Verification items for the finished model (mm, model axes). Face numbers are marked on the shaded views. A direction names the side the tool comes from. Round coordinates to 2 decimals unless told otherwise and drop trailing zeros. Loops run counter-clockwise (first coordinate to the right, second up) from the corner with the lowest first, then second, coordinate; pieces in that order, holes last. Notation, with made-up numbers: (-15, 26.5) - (17, 26.5) arc R6 ccw to (17, 32.5) - close; hole circle Ø7 at (-20, -0.5). An arc over 180 degrees is marked (long way). Use CSV: the item, a comma, the result in double quotes.
```python
from build123d import *

# Parameters (mm, degrees)
SKETCH1_R           = 3.3
BOSS_EXTRUDE1_DEPTH = 10
CUT_EXTRUDE1_DEPTH  = 5


with BuildPart() as part:
    # Sketch1 → Boss-Extrude1 (new body)
    with BuildSketch(Plane(origin=(0, 0, 0), x_dir=(1, 0, 0), z_dir=(0, 1, 0))):
        with BuildLine():
            Line((10, 0), (10, -10))
            ThreePointArc((10, -10), (0, -20), (-10, -10))
            Line((-10, -10), (-10, 0))
            ThreePointArc((-10, 0), (0, 10), (10, 0))
        make_face()
        with Locations(Location((0, 0, 0), (0, 0, 270))):
            Circle(SKETCH1_R, mode=Mode.SUBTRACT)
    extrude(amount=BOSS_EXTRUDE1_DEPTH)

    # Sketch2 → Cut-Extrude1 (cut)
    with BuildSketch(Plane.XZ):
        Polygon((6.5, 3.75277675), (0, 7.505553499), (-6.5, 3.75277675), (-6.5, -3.75277675), (0, -7.505553499), (6.5, -3.75277675), align=None)
    extrude(amount=-CUT_EXTRUDE1_DEPTH, mode=Mode.SUBTRACT)


solid = part.part
```
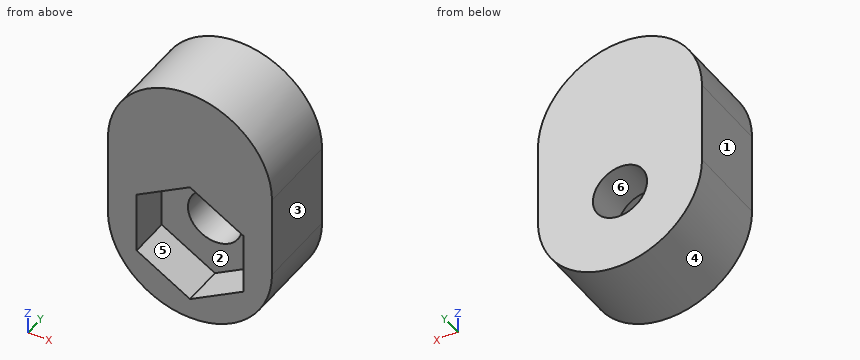
1) Access from +Z, -Z, +X, -X, +Y, -Y to the whole of each face (thin tool, end or side, straight path). Record for the marked faces 5 and 6.
Returned:
face 5,"-Y"
face 6,"+Y, -Y"
2) Mould release check, pull along X, two halves, no side actions. Record for the marked faces 1, 2, 3 and 4: +X half, -X half, draft (parallel to the pull), parting line (faces both ways), or undercut.
Returned:
face 1,"-X half"
face 2,"undercut"
face 3,"+X half"
face 4,"parting line"
3) Cross-section at D-D, the plane x = 4.25. Record the cut outline in (y, z), then the cut area to 3 significant figures.
Returned:
outline,"(0, -9.05) - (10, -9.05) - (10, 19.05) - (0, 19.05) - (0, 5.05) - (5, 5.05) - (5, -5.05) - (0, -5.05) - close"
area,"231 mm²"
4) Thickness scan on probe 1 along X at (y, z) = (6, 0); probe 2 along Z at (x, y) = (0, 8.7); probe 3 along Y at (x, z) = (0.75, -6). Record the ranges inside material, lowest first. Write a range as [from, to].
Returned:
probe 1,"x = [-10, -3.3], [3.3, 10]"
probe 2,"z = [-10, -3.3], [3.3, 20]"
probe 3,"y = [5, 10]"
5) Cross-section at A-A, the plane y = 3.75. Record the cut outline in (x, z).
Returned:
outline,"(-10, 0) arc R10 ccw to (10, 0) - (10, 10) arc R10 ccw to (-10, 10) - close; hole (-6.5, -3.75) - (0, -7.51) - (6.5, -3.75) - (6.5, 3.75) - (0, 7.51) - (-6.5, 3.75) - close"
6) Cross-section at B-B, the plane x = -2.5. Record the cut outline in (y, z), then the cut area to 3 significant figures.
Returned:
outline,"(0, -9.68) - (10, -9.68) - (10, -2.15) - (5, -2.15) - (5, -6.06) - (0, -6.06) - close; (0, 6.06) - (5, 6.06) - (5, 2.15) - (10, 2.15) - (10, 19.68) - (0, 19.68) - close"
area,"211 mm²"
7) Gauge pin test, flat ends, axial feed: pin 1 Ø5 at (x, z) = (-2, 14.5) entering from -Y; pin 2 Ø7.5 at (x, z) = (0, 0) entering from -Y; pin 3 Ø1 at (y, z) = (6.5, 13.5) entering from -X; pin 4 Ø4 at (y, z) = (6.5, -3.5) entering from +X. Record the tip position at first contact, or that the pin passes through.
Returned:
pin 1,"stops at y = 0"
pin 2,"stops at y = 5"
pin 3,"stops at x = -9.54"
pin 4,"stops at x = 9.89"
8) Cross-section at C-C, the plane z = 7. Record the cut outline in (x, y).
Returned:
outline,"(-10, 0) - (-0.88, 0) - (-0.88, 5) - (0.88, 5) - (0.88, 0) - (10, 0) - (10, 10) - (-10, 10) - close"
